Could you check a few things on this model? Use its own coordinates, in mm. A direction names the side the tool comes from. Coordinates: 2 decimals unless noted, no trailing zeros. Loops run counter-clockwise (first coordinate to the right, second up) from the corner with the lowest first, then second, coordinate; pieces in that order, holes last.
from build123d import *

# Parameters (mm, degrees)
SKETCH_W        = 48
SKETCH_H        = 28
PAD_DEPTH       = 8
POCKET_DEPTH    = 6
SKETCH002_W     = 4
SKETCH002_H     = 8
POCKET001_DEPTH = 5
SKETCH004_R     = 1.2
POCKET002_DEPTH = 3


with BuildPart() as part:
    # Sketch → Pad (new body)
    with BuildSketch(Plane.XY):
        with Locations((24, 14)):
            Rectangle(SKETCH_W, SKETCH_H)
    extrude(amount=PAD_DEPTH)

    # Sketch001 → Pocket (cut)
    with BuildSketch(Plane.XY.offset(8)):
        with BuildLine():
            Line((3.5, 3.2), (7.7, 3.2))
            Line((7.7, 3.2), (7.7, 4.4))
            ThreePointArc((8.3, 4.4), (8, 4.7), (7.7, 4.4))
            Line((8.3, 4.4), (8.3, 3.2))
            Line((8.3, 3.2), (33.4, 3.2))
            Line((33.4, 3.2), (33.4, 4.4))
            ThreePointArc((34, 4.4), (33.7, 4.7), (33.4, 4.4))
            Line((34, 4.4), (34, 3.2))
            Line((34, 3.2), (44.5, 3.2))
            Line((44.5, 3.2), (44.5, 24.8))
            Line((44.5, 24.8), (34, 24.8))
            Line((34, 24.8), (34, 23.6))
            ThreePointArc((33.4, 23.6), (33.7, 23.3), (34, 23.6))
            Line((33.4, 23.6), (33.4, 24.8))
            Line((33.4, 24.8), (8.3, 24.8))
            Line((8.3, 24.8), (8.3, 23.6))
            ThreePointArc((7.7, 23.6), (8, 23.3), (8.3, 23.6))
            Line((7.7, 23.6), (7.7, 24.8))
            Line((7.7, 24.8), (3.5, 24.8))
            Line((3.5, 24.8), (3.5, 3.2))
        make_face()
    extrude(amount=-POCKET_DEPTH, mode=Mode.SUBTRACT)

    # Sketch002 → Pocket001 (cut)
    with BuildSketch(Plane.XY.offset(8)):
        with Locations((2, 14)):
            Rectangle(SKETCH002_W, SKETCH002_H)
    extrude(amount=-POCKET001_DEPTH, mode=Mode.SUBTRACT)

    # Sketch004 → Pocket002 (cut)
    with BuildSketch(Plane.XY.offset(8)):
        with Locations((1.8, 26.2)):
            Circle(SKETCH004_R)
        with Locations((1.8, 1.8)):
            Circle(SKETCH004_R)
        with Locations((46.2, 1.382931)):
            Circle(SKETCH004_R)
        with Locations((46.2, 26.2)):
            Circle(SKETCH004_R)
    extrude(amount=-POCKET002_DEPTH, mode=Mode.SUBTRACT)


solid = part.part
(1) Imagine slicing it at B-B, the plane y = 26.2. Write out the boundary of the cut face in (x, z).
Answers:
outline: (0, 0) - (48, 0) - (48, 8) - (47.4, 8) - (47.4, 5) - (45, 5) - (45, 8) - (3, 8) - (3, 5) - (0.6, 5) - (0.6, 8) - (0, 8) - close
(2) Imagine slicing it at C-C, the plane z = 7.25. State how many separate pieces and enclosed holes the cut face has, and give its area (3 significant figures).
Answers:
separate pieces: 1
enclosed holes: 4
area: 416 mm2
(3) I need wall thicknesses on probe 1 along Y at (x, z) = (46.2, 5.8); probe 2 along Y at (x, z) = (23, 6); probe 3 along X at (y, z) = (8.5, 4). Which ranges of each line are inside material? Lowest first, please.
Answers:
probe 1: y = 0 to 0.18, 2.58 to 25, 27.4 to 28
probe 2: y = 0 to 3.2, 24.8 to 28
probe 3: x = 0 to 3.5, 44.5 to 48
(4) We'd pull the mould along Y, two halves only. Please class faces 1 (the face through (24, 0, 4)), 2 (the face through (24, 28, 4)), 3 (the face through (2, 2, 5)): +Y half, -Y half, draft (parallel to the pull), parting line (faces both ways), or undercut.
Answers:
face 1: -Y half
face 2: +Y half
face 3: undercut
(5) For pin 1 (3 mm diameter, centred on x = 1.8, y = 1.8, fed in from +Z); pin 2 (10 mm diameter, centred on x = 37.5, y = 9.5, fed in from +Z); pin 3 (0.7 mm diameter, centred on x = 2, y = 2, fed in from +Z), each with a flat end and sliding along its axis, tell me the tip position at first contact or that it passes through.
Answers:
pin 1: stops at z = 8
pin 2: stops at z = 2
pin 3: stops at z = 5
(6) Imagine slicing it at A-A, the plane x = 46.2. Write out the boundary of the cut face in (y, z), and give its area (3 significant figures).
Answers:
outline: (0, 0) - (28, 0) - (28, 8) - (27.4, 8) - (27.4, 5) - (25, 5) - (25, 8) - (2.58, 8) - (2.58, 5) - (0.18, 5) - (0.18, 8) - (0, 8) - close
area: 210 mm2
(7) Imagine slicing it at D-D, the plane z = 4.5. Write out the boundary of the cut face in (x, y).
Answers:
outline: (0, 0) - (48, 0) - (48, 28) - (0, 28) - (0, 18) - (3.5, 18) - (3.5, 24.8) - (7.7, 24.8) - (7.7, 23.6) arc R0.3 ccw to (8.3, 23.6) - (8.3, 24.8) - (33.4, 24.8) - (33.4, 23.6) arc R0.3 ccw to (34, 23.6) - (34, 24.8) - (44.5, 24.8) - (44.5, 3.2) - (34, 3.2) - (34, 4.4) arc R0.3 ccw to (33.4, 4.4) - (33.4, 3.2) - (8.3, 3.2) - (8.3, 4.4) arc R0.3 ccw to (7.7, 4.4) - (7.7, 3.2) - (3.5, 3.2) - (3.5, 10) - (0, 10) - close
(8) Which directions (+Z, -Z, +X, -X, +Y, -Y) give clear straight access to the entire face, cutting with the end or side of a thin tool? Please do faces 4 (the face through (24, 14, 0)), 5 (the face through (34, 4, 5)), 6 (the face through (2, 14, 3)).
Answers:
face 4: -Z, +X, -X, +Y, -Y
face 5: +Z
face 6: +Z, -X
